Work out the finished part from the listing and answer in its coordinate system (mm). A direction names the side the tool comes from. Give positions to 0.01 mm unless a question says otherwise; leave off trailing zeros. Order: outer loops, then holes, each group sorted by start corner. A loop starts at its lowest first (then second) coordinate and runs counter-clockwise, first axis right, second up. Notation, with made-up numbers: (-24.5, -21.75) -> (19.5, -21.75) arc R13 ccw to (19.5, -5.75) -> close; hole circle Ø10 at (-11.5, 57). An arc over 180 degrees is marked (long way). Answer as CSV lines item,"result". Start each with the question number.
1. A cutting plane is placed at B-B (y = 10.5). State how many separate pieces and enclosed holes the cut face has, then the cut area to 3 significant figures.
2. Flat-ended cylindrical pins translate along their axes: pin 1 (17 mm diameter, centred on x = -127, z = 0, fed in from +Y); pin 2 (8 mm diameter, centred on x = -92, z = 92, fed in from +Y); pin 3 (8 mm diameter, centred on x = 325.5, y = 15, fed in from +Z); pin 4 (5.5 mm diameter, centred on x = -96, z = 72, fed in from +Y). Find the tip coordinate at first contact, or state that the pin passes through.
3. For a pull along X with two mould halves and no side action, classify faces 1 (the cylindrical face through (136.516, 12.209, -0.419)), 2 (the flat face through (-457.2, 13, 0)), 3 (the flat face through (-6, 13, -38.1)) as released by +X, released by -X, zero draft, split by the parting line, or undercut.
4. A cutting plane is placed at C-C (x = -233). Give the vertices of the cut face in (y, z).
5. A cutting plane is placed at A-A (x = 127). Give the vertices of the cut face in (y, z) (3 decimals), then the cut area to 3 significant figures.
6. Find the intervals of material crossed by L1, parallel to X at y = 7, z = 69.85; L2, parallel to X at y = 19.5, z = 69.85; L3, parallel to Z at x = -50.8, y = 8, in increasing order.
7. For faces 4 (the flat face through (-2, 22.86, 66)), 5 (the flat face through (12.7, 11, 125)), 6 (the flat face through (-67, 11, 88.9)), determine the directions among +Z, -Z, +X, -X, +Y, -Y from which every point of the face is accessible in a straight line to the end or side of a thin tool.
from build123d import *

# Parameters (mm, degrees)
SKETCH1_W                                        = 914.4
SKETCH1_H                                        = 76.2
BOSS_EXTRUDE1_DEPTH                              = 25.4
FILLET1_R                                        = 6.35
F_3_4_0_7500_DOWEL_HOLE1_D                       = 19.05
F_3_4_0_7500_DOWEL_HOLE1_CSINK_D                 = 20.32
F_3_4_0_7500_DOWEL_HOLE1_CSINK_ANGLE             = 90
BOSS_EXTRUDE2_DEPTH                              = 22.86
FILLET2_R                                        = 6.35
F_5_16_18_TAPPED_HOLE1_D                         = 6.5278
F_1_2_13_TAPPED_HOLE1_D                          = 10.71626
F_1_2_13_TAPPED_HOLE1_CSINK_D                    = 13.97
F_1_2_13_TAPPED_HOLE1_CSINK_ANGLE                = 90
CBORE_FOR_1_4_SOCKET_HEAD_CAP_SCREW1_D           = 6.7564
CBORE_FOR_1_4_SOCKET_HEAD_CAP_SCREW1_CBORE_D     = 11.1125
CBORE_FOR_1_4_SOCKET_HEAD_CAP_SCREW1_CBORE_DEPTH = 6.35


with BuildPart() as part:
    # Sketch1 → Boss-Extrude1 (new body)
    with BuildSketch(Plane(origin=(0, 0, 0), x_dir=(1, 0, 0), z_dir=(0, 1, 0))):
        Rectangle(SKETCH1_W, SKETCH1_H)
    extrude(amount=BOSS_EXTRUDE1_DEPTH)

    # Fillet1
    fillet1_edges = [part.edges().sort_by_distance(p)[0] for p in [
        (457.2, 12.7, 38.1),
        (-457.2, 12.7, 38.1),
        (-457.2, 12.7, -38.1),
        (457.2, 12.7, -38.1),
    ]]
    fillet(fillet1_edges, radius=FILLET1_R)

    # 3/4 (0.7500) Dowel Hole1 (through all)
    with Locations(Plane(origin=(0, 25.4, 0), x_dir=(1, 0, 0), z_dir=(0, 1, 0))):
        with Locations((-127, 0), (127, 0)):
            CounterSinkHole(F_3_4_0_7500_DOWEL_HOLE1_D / 2, F_3_4_0_7500_DOWEL_HOLE1_CSINK_D / 2, counter_sink_angle=F_3_4_0_7500_DOWEL_HOLE1_CSINK_ANGLE)

    # Sketch7 → Boss-Extrude2 (add)
    with BuildSketch(Plane(origin=(0, 0, 0), x_dir=(1, 0, 0), z_dir=(0, 1, 0))):
        Polygon((-27.364696837, -88.9), (-12.7, -114.3), (-12.7, -139.7), (12.7, -139.7), (12.7, -114.3), (27.364696837, -88.9), (107.95, -88.9), (107.95, -38.1), (-107.95, -38.1), (-107.95, -88.9), align=None)
    extrude(amount=BOSS_EXTRUDE2_DEPTH)

    # Fillet2
    fillet2_edges = [part.edges().sort_by_distance(p)[0] for p in [
        (107.95, 11.43, 88.9),
        (107.95, 11.43, 38.1),
        (-107.95, 11.43, 38.1),
        (-107.95, 11.43, 88.9),
        (-27.364696837, 11.43, 88.9),
        (-12.7, 11.43, 114.3),
        (-12.7, 11.43, 139.7),
        (12.7, 11.43, 139.7),
        (12.7, 11.43, 114.3),
        (27.364696837, 11.43, 88.9),
    ]]
    fillet(fillet2_edges, radius=FILLET2_R)

    # 5/16-18 Tapped Hole1 (through all)
    with Locations(Plane(origin=(0, 0, 0), x_dir=(-1, 0, 0), z_dir=(0, -1, 0))):
        with Locations((0, -127)):
            Hole(F_5_16_18_TAPPED_HOLE1_D / 2)

    # 1/2-13 Tapped Hole1 (through all)
    with Locations(Plane(origin=(0, 25.4, 0), x_dir=(1, 0, 0), z_dir=(0, 1, 0))):
        with Locations((-50.8, 0), (50.8, 0)):
            CounterSinkHole(F_1_2_13_TAPPED_HOLE1_D / 2, F_1_2_13_TAPPED_HOLE1_CSINK_D / 2, counter_sink_angle=F_1_2_13_TAPPED_HOLE1_CSINK_ANGLE)

    # CBORE for 1/4 Socket Head Cap Screw1 (through all)
    with Locations(Plane(origin=(0, 22.86, 0), x_dir=(1, 0, 0), z_dir=(0, 1, 0))):
        with Locations((-95.25, -69.85), (95.25, -69.85)):
            CounterBoreHole(CBORE_FOR_1_4_SOCKET_HEAD_CAP_SCREW1_D / 2, CBORE_FOR_1_4_SOCKET_HEAD_CAP_SCREW1_CBORE_D / 2, CBORE_FOR_1_4_SOCKET_HEAD_CAP_SCREW1_CBORE_DEPTH)


solid = part.part
Answer sheet:
1,separate pieces,"1"
1,enclosed holes,"7"
1,area,"81,400 mm^2"
2,pin 1,"passes through"
2,pin 2,"stops at y = 22.86"
2,pin 3,"stops at z = 38.1"
2,pin 4,"stops at y = 16.51"
3,face 1,"undercut"
3,face 2,"released by -X"
3,face 3,"zero draft"
4,outline,"(0, -38.1) -> (25.4, -38.1) -> (25.4, 38.1) -> (0, 38.1) -> close"
5,outline,"(0, -38.1) -> (25.4, -38.1) -> (25.4, -10.16) -> (24.765, -9.525) -> (0, -9.525) -> close; (0, 9.525) -> (24.765, 9.525) -> (25.4, 10.16) -> (25.4, 38.1) -> (0, 38.1) -> close"
5,area,"1,450 mm^2"
6,L1,"x = -107.95 to -98.63, -91.87 to 91.87, 98.63 to 107.95"
6,L2,"x = -107.95 to -100.81, -89.69 to 89.69, 100.81 to 107.95"
6,L3,"z = -38.1 to -5.36, 5.36 to 88.9"
7,face 4,"+Z, +X, -X, +Y"
7,face 5,"+Z, +X, +Y, -Y"
7,face 6,"+Z, -X, +Y, -Y"
